```python
from build123d import *

# Parameters (mm, degrees)
F0_W     = 50.8
F0_H     = 101.6
F1_DEPTH = 3.175


with BuildPart() as f1:
    # F0 (on Front) → F1 (new body)
    with BuildSketch(Plane.XZ):
        Polygon((-254, 0), (0, 0), (0, 50.8), (-203.2, 50.8), (-254, 50.8), align=None)
        with Locations((-228.6, 101.6)):
            Rectangle(F0_W, F0_H)
        Polygon((-254, 203.2), (-254, 152.4), (-203.2, 152.4), (0, 152.4), (0, 203.2), (-50.8, 203.2), align=None)
        with Locations((-25.4, 254)):
            Rectangle(F0_W, F0_H)
        Polygon((-254, 304.8), (-50.8, 304.8), (0, 304.8), (0, 355.6), (-254, 355.6), align=None)
    extrude(amount=-F1_DEPTH)


solid = f1.part
```
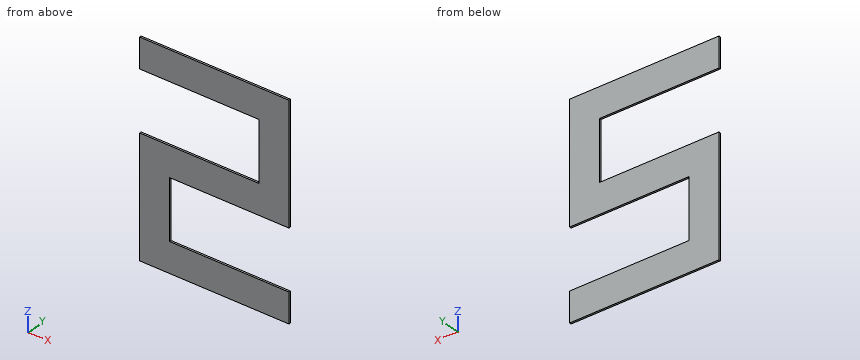
Geometry: final body of the model. Coordinates: model frame, mm. Give positions to 0.01 mm unless a question says otherwise; leave off trailing zeros. Loops run counter-clockwise (first coordinate to the right, second up) from the corner with the lowest first, then second, coordinate; pieces in that order, holes last. Notation, with made-up numbers: (5, 64) - (26, 64) arc R17 cw to (26, 86) - close; hole circle Ø5 at (-30, 65). An arc over 180 degrees is marked (long way). Answer as CSV lines item,"result". Start each with the question number.
(1) Section query A-A (x = -229). Output: boundary loops of the cut face in (y, z) (3 decimals), and give its area (3 significant figures).
(2) Section query B-B (x = -64). Output: boundary loops of the cut face in (y, z) (3 decimals).
(3) Pin query (flat end, axial travel): P1, Ø1.6, axis at y = 2, z = 114.5, coming from the +X side; P2, Ø1, axis at y = 1, z = 244, coming from the -X side. Return the tip coordinate at first contact, or that it passes through.
(4) Ray query, line 1 along Z through (x, y) = (-79.5, 2.8); line 2 along Z through (x, y) = (-215.5, 1.2); line 3 along Z through (x, y) = (-36.5, 2.6). Return the intervals inside material, ascending. Write a range as [from, to].
(5) Section query C-C (y = 2.2). Output: boundary loops of the cut face in (x, z), and give its area (3 significant figures).
(6) Section query D-D (z = 222). Output: boundary loops of the cut face in (x, y) (3 decimals), and give its area (3 significant figures).
Worked answers:
1,outline,"(0, 0) - (3.175, 0) - (3.175, 203.2) - (0, 203.2) - close; (0, 304.8) - (3.175, 304.8) - (3.175, 355.6) - (0, 355.6) - close"
1,area,"806 mm^2"
2,outline,"(0, 0) - (3.175, 0) - (3.175, 50.8) - (0, 50.8) - close; (0, 152.4) - (3.175, 152.4) - (3.175, 203.2) - (0, 203.2) - close; (0, 304.8) - (3.175, 304.8) - (3.175, 355.6) - (0, 355.6) - close"
3,P1,"stops at x = -203.2"
3,P2,"stops at x = -50.8"
4,line 1,"z = [0, 50.8], [152.4, 203.2], [304.8, 355.6]"
4,line 2,"z = [0, 203.2], [304.8, 355.6]"
4,line 3,"z = [0, 50.8], [152.4, 355.6]"
5,outline,"(-254, 0) - (0, 0) - (0, 50.8) - (-203.2, 50.8) - (-203.2, 152.4) - (0, 152.4) - (0, 355.6) - (-254, 355.6) - (-254, 304.8) - (-50.8, 304.8) - (-50.8, 203.2) - (-254, 203.2) - close"
5,area,"49,000 mm^2"
6,outline,"(-50.8, 0) - (0, 0) - (0, 3.175) - (-50.8, 3.175) - close"
6,area,"161 mm^2"
